For this review, take the finished solid that the model builds, in its own axes (mm). Face numbers are marked on the shaded views. A direction names the side the tool comes from. Coordinates: 2 decimals unless noted, no trailing zeros. Write each loop counter-clockwise with the first axis right and the second up, starting at its lowest first coordinate (ties: lowest second). Pieces come first, ordered by that corner, then holes. Notation, with made-up numbers: (20.5, 80.25) -> (78.5, 80.25) arc R28 cw to (78.5, 100.25) -> close; hole circle Ø5 at (37, 60). An arc over 180 degrees is marked (long way). Put each result on its own line as item: value. Start each with the question number.
Item 1: To check wall thickness, follow L1, parallel to Y at x = 10, z = 15; L2, parallel to X at y = -22, z = 14; L3, parallel to Z at x = 10, y = -5.5. State the ranges of each line that lie inside material, in increasing order.
Item 2: Consider section A-A on y = -22.5. Give the boundary of the cut face in (x, z), and give its area (3 significant figures).
Item 3: Consider section C-C on y = 5. Give the number of separate pieces and of enclosed holes in the cut face, and give its area (3 significant figures).
Item 4: Insertion check: P1, Ø1, axis at x = 4.5, z = 2.5, coming from the -Y side; P2, Ø5.5, axis at x = 25, y = -22.5, coming from the -Z side; P3, Ø6, axis at x = 20.5, z = -2.5, coming from the -Y side. Each pin has a flat end and moves straight along its axis. Give the tip position at first contact, or say it passes through.
Item 5: The part is to be moulded in two halves that separate along Z. For the marked faces 3, 4, 5 and 6, say which applies: +Z half, -Z half, draft (parallel to the pull), parting line (faces both ways), or undercut.
Item 6: For the marked faces 1 and 2, list the 3-axis set-ups (+Z, -Z, +X, -X, +Y, -Y) from which the entire face can be reached by the end or side of a thin tool; tool diameter is ignored.
Item 7: Consider section B-B on z = -18. Give the boundary of the cut face in (x, y), and give its area (3 significant figures).
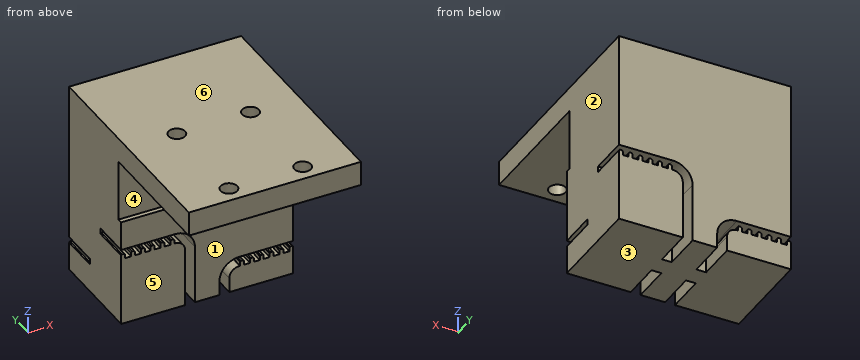
```python
from build123d import *

# Parameters (mm, degrees)
SKETCH1_W           = 35
SKETCH1_H           = 22
BOSS_EXTRUDE1_DEPTH = 20
CUT_EXTRUDE1_DEPTH  = 8
CUT_EXTRUDE2_DEPTH  = 8
BOSS_EXTRUDE2_DEPTH = 8
BOSS_EXTRUDE4_DEPTH = 8
SKETCH9_W           = 35
SKETCH9_H           = 19
BOSS_EXTRUDE5_DEPTH = 12.5
SKETCH11_W          = 35
SKETCH11_H          = 46
BOSS_EXTRUDE6_DEPTH = 5
SKETCH12_R          = 1.7
CUT_EXTRUDE3_DEPTH  = 5


with BuildPart() as part:
    # Sketch1 → Boss-Extrude1 (new body)
    with BuildSketch(Plane(origin=(0, 0, 0), x_dir=(1, 0, 0), z_dir=(0, 1, 0))):
        with Locations((17.5, 11)):
            Rectangle(SKETCH1_W, SKETCH1_H)
    extrude(amount=BOSS_EXTRUDE1_DEPTH)

    # Sketch2 → Cut-Extrude1 (cut)
    with BuildSketch(Plane(origin=(0, 20, 0), x_dir=(1, 0, 0), z_dir=(0, 1, 0))):
        with BuildLine():
            Line((0, 15), (11, 15))
            ThreePointArc((11, 15), (13.828427125, 16.171572875), (15, 19))
            Line((15, 19), (15, 22))
            Line((15, 22), (13, 22))
            Line((13, 22), (13, 19))
            ThreePointArc((13, 19), (12.414213562, 17.585786438), (11, 17))
            Line((11, 17), (0, 17))
            Line((0, 17), (0, 15))
        make_face()
        with BuildLine():
            Line((35, 6), (24, 6))
            ThreePointArc((24, 6), (21.171572875, 7.171572875), (20, 10))
            Line((20, 10), (20, 22))
            Line((20, 22), (22, 22))
            Line((22, 22), (22, 10))
            ThreePointArc((22, 10), (22.585786438, 8.585786438), (24, 8))
            Line((24, 8), (35, 8))
            Line((35, 8), (35, 6))
        make_face()
    extrude(amount=-CUT_EXTRUDE1_DEPTH, mode=Mode.SUBTRACT)

    # Sketch5 → Cut-Extrude2 (cut)
    with BuildSketch(Plane(origin=(0, 0, 0), x_dir=(-1, 0, 0), z_dir=(0, -1, 0))):
        with BuildLine():
            Line((-35, 15), (-24, 15))
            ThreePointArc((-24, 15), (-21.171572875, 16.171572875), (-20, 19))
            Line((-20, 19), (-20, 22))
            Line((-20, 22), (-22, 22))
            Line((-22, 22), (-22, 19))
            ThreePointArc((-22, 19), (-22.585786438, 17.585786438), (-24, 17))
            Line((-24, 17), (-35, 17))
            Line((-35, 17), (-35, 15))
        make_face()
        with BuildLine():
            Line((0, 6), (-11, 6))
            ThreePointArc((-11, 6), (-13.828427125, 7.171572875), (-15, 10))
            Line((-15, 10), (-15, 22))
            Line((-15, 22), (-13, 22))
            Line((-13, 22), (-13, 10))
            ThreePointArc((-13, 10), (-12.414213562, 8.585786438), (-11, 8))
            Line((-11, 8), (0, 8))
            Line((0, 8), (0, 6))
        make_face()
    extrude(amount=-CUT_EXTRUDE2_DEPTH, mode=Mode.SUBTRACT)

    # Sketch6 → Boss-Extrude2 (add)
    with BuildSketch(Plane(origin=(0, 20, 0), x_dir=(1, 0, 0), z_dir=(0, 1, 0))):
        Polygon((0.2, 16), (0, 16.2), (0, 17), (0.8, 17), (0.8, 16.2), (0.6, 16), align=None)
        Polygon((2.2, 16), (2, 16.2), (2, 17), (2.8, 17), (2.8, 16.2), (2.6, 16), align=None)
        Polygon((4.2, 16), (4, 16.2), (4, 17), (4.8, 17), (4.8, 16.2), (4.6, 16), align=None)
        Polygon((6.2, 16), (6, 16.2), (6, 17), (6.8, 17), (6.8, 16.2), (6.6, 16), align=None)
        Polygon((8.2, 16), (8, 16.2), (8, 17), (8.8, 17), (8.8, 16.2), (8.6, 16), align=None)
        Polygon((10.2, 16), (10, 16.2), (10, 17), (10.8, 17), (10.8, 16.2), (10.6, 16), align=None)
        Polygon((34.4, 7), (34.2, 7.2), (34.2, 8), (35, 8), (35, 7.2), (34.8, 7), align=None)
        Polygon((32.4, 7), (32.2, 7.2), (32.2, 8), (33, 8), (33, 7.2), (32.8, 7), align=None)
        Polygon((30.4, 7), (30.2, 7.2), (30.2, 8), (31, 8), (31, 7.2), (30.8, 7), align=None)
        Polygon((28.4, 7), (28.2, 7.2), (28.2, 8), (29, 8), (29, 7.2), (28.8, 7), align=None)
        Polygon((26.4, 7), (26.2, 7.2), (26.2, 8), (27, 8), (27, 7.2), (26.8, 7), align=None)
        Polygon((24.4, 7), (24.2, 7.2), (24.2, 8), (25, 8), (25, 7.2), (24.8, 7), align=None)
    extrude(amount=-BOSS_EXTRUDE2_DEPTH)

    # Sketch8 → Boss-Extrude4 (add)
    with BuildSketch(Plane.XZ):
        Polygon((35, -17), (35, -16.2), (34.8, -16), (34.4, -16), (34.2, -16.2), (34.2, -17), align=None)
        Polygon((33, -17), (33, -16.2), (32.8, -16), (32.4, -16), (32.2, -16.2), (32.2, -17), align=None)
        Polygon((31, -17), (31, -16.2), (30.8, -16), (30.4, -16), (30.2, -16.2), (30.2, -17), align=None)
        Polygon((29, -17), (29, -16.2), (28.8, -16), (28.4, -16), (28.2, -16.2), (28.2, -17), align=None)
        Polygon((27, -17), (27, -16.2), (26.8, -16), (26.4, -16), (26.2, -16.2), (26.2, -17), align=None)
        Polygon((25, -17), (25, -16.2), (24.8, -16), (24.4, -16), (24.2, -16.2), (24.2, -17), align=None)
        Polygon((0.8, -8), (0.8, -7.2), (0.6, -7), (0.2, -7), (0, -7.2), (0, -8), align=None)
        Polygon((2.8, -8), (2.8, -7.2), (2.6, -7), (2.2, -7), (2, -7.2), (2, -8), align=None)
        Polygon((4.8, -8), (4.8, -7.2), (4.6, -7), (4.2, -7), (4, -7.2), (4, -8), align=None)
        Polygon((6.8, -8), (6.8, -7.2), (6.6, -7), (6.2, -7), (6, -7.2), (6, -8), align=None)
        Polygon((8.8, -8), (8.8, -7.2), (8.6, -7), (8.2, -7), (8, -7.2), (8, -8), align=None)
        Polygon((10.8, -8), (10.8, -7.2), (10.6, -7), (10.2, -7), (10, -7.2), (10, -8), align=None)
    extrude(amount=-BOSS_EXTRUDE4_DEPTH)

    # Sketch9 → Boss-Extrude5 (add)
    with BuildSketch(Plane.XY):
        with Locations((17.5, 10.5)):
            Rectangle(SKETCH9_W, SKETCH9_H)
    extrude(amount=BOSS_EXTRUDE5_DEPTH)

    # Sketch11 → Boss-Extrude6 (add)
    with BuildSketch(Plane.XY.offset(12.5)):
        with Locations((17.5, -3)):
            Rectangle(SKETCH11_W, SKETCH11_H)
    extrude(amount=BOSS_EXTRUDE6_DEPTH)

    # Sketch12 → Cut-Extrude3 (cut)
    with BuildSketch(Plane.XY.offset(17.5)):
        with Locations((10, -2.5)):
            Circle(SKETCH12_R)
        with Locations((25, -2.5)):
            Circle(SKETCH12_R)
        with Locations((25, -22.5)):
            Circle(SKETCH12_R)
        with Locations((10, -22.5)):
            Circle(SKETCH12_R)
    extrude(amount=-CUT_EXTRUDE3_DEPTH, mode=Mode.SUBTRACT)


solid = part.part
```
Return value:
1. L1: -26 to -24.2, -20.8 to -4.2, -0.8 to 20
1. L2: 0 to 8.38, 11.62 to 23.38, 26.62 to 35
1. L3: 12.5 to 17.5
2. outline: (0, 12.5) -> (8.3, 12.5) -> (8.3, 17.5) -> (0, 17.5) -> close; (11.7, 12.5) -> (23.3, 12.5) -> (23.3, 17.5) -> (11.7, 17.5) -> close; (26.7, 12.5) -> (35, 12.5) -> (35, 17.5) -> (26.7, 17.5) -> close
2. area: 141 mm^2
3. separate pieces: 3
3. enclosed holes: 0
3. area: 1,300 mm^2
4. P1: y = 1
4. P2: z = 12.5
4. P3: y = 0
5. face 3: -Z half
5. face 4: undercut
5. face 5: draft
5. face 6: +Z half
6. face 1: -Z, +X, -X, -Y
6. face 2: +Z, -Z, +X, +Y, -Y
7. outline: (0, 0) -> (13, 0) -> (13, 8) -> (15, 8) -> (15, 0) -> (20.13, 0) -> (20.13, 8) -> (22.27, 8) -> (22.27, 0) -> (35, 0) -> (35, 20) -> (22, 20) -> (22, 12) -> (20, 12) -> (20, 20) -> (14.87, 20) -> (14.87, 12) -> (12.73, 12) -> (12.73, 20) -> (0, 20) -> close
7. area: 634 mm^2
